Read the model definition and answer for the solid it produces. Units are mm, in the model's axes. A direction names the side the tool comes from. Coordinates: 2 decimals unless noted, no trailing zeros. Loops run counter-clockwise (first coordinate to the right, second up) from the corner with the lowest first, then second, coordinate; pieces in that order, holes last.
from build123d import *

# Parameters (mm, degrees)
ESBO_O1_W                = 400
ESBO_O1_H                = 150
RESSALTO_EXTRUS_O1_DEPTH = 9
ESBO_O2_W                = 10
ESBO_O2_H                = 150
RESSALTO_EXTRUS_O2_DEPTH = 450
ESBO_O5_R                = 35
CORTE_EXTRUS_O1_DEPTH    = 300
ESBO_O6_W                = 400
ESBO_O6_H                = 10
RESSALTO_EXTRUS_O4_DEPTH = 230
ESBO_O8_W                = 100
ESBO_O8_H                = 50
RESSALTO_EXTRUS_O5_DEPTH = 25
ESBO_O9_R                = 5
CORTE_EXTRUS_O3_DEPTH    = 50
ESBO_O7_R                = 5
CORTE_EXTRUS_O2_DEPTH    = 150
ESBO_O11_W               = 100
ESBO_O11_H               = 50
RESSALTO_EXTRUS_O6_DEPTH = 50
ESBO_O12_R               = 5
CORTE_EXTRUS_O4_DEPTH    = 30
ESBO_O13_W               = 44
ESBO_O13_H               = 45
ESBO_O13_H_2             = 44
CORTE_EXTRUS_O5_DEPTH    = 100
ESBO_O14_R               = 5
CORTE_EXTRUS_O6_DEPTH    = 10


with BuildPart() as part:
    # Esboço1 → Ressalto-extrusão1 (new body)
    with BuildSketch(Plane(origin=(0, 0, 0), x_dir=(1, 0, 0), z_dir=(0, 1, 0))):
        Rectangle(ESBO_O1_W, ESBO_O1_H)
    extrude(amount=RESSALTO_EXTRUS_O1_DEPTH)

    # Esboço2 → Ressalto-extrusão2 (add)
    with BuildSketch(Plane(origin=(0, 9, 0), x_dir=(1, 0, 0), z_dir=(0, 1, 0))):
        with Locations((-126, 0)):
            Rectangle(ESBO_O2_W, ESBO_O2_H)
        with Locations((126, 0)):
            Rectangle(ESBO_O2_W, ESBO_O2_H)
    extrude(amount=RESSALTO_EXTRUS_O2_DEPTH)

    # Esboço5 → Corte-extrusão1 (cut)
    with BuildSketch(Plane.ZY.offset(131)):
        with Locations((0, 359)):
            Circle(ESBO_O5_R)
    extrude(amount=-CORTE_EXTRUS_O1_DEPTH, mode=Mode.SUBTRACT)

    # Esboço6 → Ressalto-extrusão4 (add)
    with BuildSketch(Plane.XZ):
        with Locations((0, 80)):
            Rectangle(ESBO_O6_W, ESBO_O6_H)
    extrude(amount=-RESSALTO_EXTRUS_O4_DEPTH)

    # Esboço8 → Ressalto-extrusão5 (add, symmetric)
    with BuildSketch(Plane.ZY):
        with Locations((135, 204)):
            Rectangle(ESBO_O8_W, ESBO_O8_H)
    extrude(amount=RESSALTO_EXTRUS_O5_DEPTH, both=True)

    # Esboço9 → Corte-extrusão3 (cut)
    with BuildSketch(Plane(origin=(0, 230, 0), x_dir=(-1, 0, 0), z_dir=(0, 1, 0))):
        with Locations(Location((0, 155, 0), (0, 0, 90))):
            Circle(ESBO_O9_R)
    extrude(amount=-CORTE_EXTRUS_O3_DEPTH, mode=Mode.SUBTRACT)

    # Esboço7 → Corte-extrusão2 (cut)
    with BuildSketch(Plane(origin=(0, 0, 75), x_dir=(-1, 0, 0), z_dir=(0, 0, -1))):
        with Locations((0, 115)):
            Circle(ESBO_O7_R)
    extrude(amount=-CORTE_EXTRUS_O2_DEPTH, mode=Mode.SUBTRACT)

    # Esboço11 → Ressalto-extrusão6 (add)
    with BuildSketch(Plane.ZY.offset(-75)):
        with Locations((135, 26)):
            Rectangle(ESBO_O11_W, ESBO_O11_H)
    extrude(amount=RESSALTO_EXTRUS_O6_DEPTH)

    # Esboço12 → Corte-extrusão4 (cut)
    with BuildSketch(Plane.ZY.offset(-25)):
        with Locations((139.811131484, 26)):
            Circle(ESBO_O12_R)
    extrude(amount=-CORTE_EXTRUS_O4_DEPTH, mode=Mode.SUBTRACT)

    # Esboço13 → Corte-extrusão5 (cut)
    with BuildSketch(Plane.XY.offset(185)):
        with Locations((50, 25.5)):
            Rectangle(ESBO_O13_W, ESBO_O13_H)
        with Locations((0, 204)):
            Rectangle(ESBO_O13_W, ESBO_O13_H_2)
    extrude(amount=-CORTE_EXTRUS_O5_DEPTH, mode=Mode.SUBTRACT)

    # Esboço14 → Corte-extrusão6 (cut)
    with BuildSketch(Plane.XY.offset(85)):
        with Locations((0, 204)):
            Circle(ESBO_O14_R)
        with Locations((50, 25.5)):
            Circle(ESBO_O14_R)
    extrude(amount=-CORTE_EXTRUS_O6_DEPTH, mode=Mode.SUBTRACT)


solid = part.part
Item 1: A cutting plane is placed at A-A on y = 387. Determine the outline of the cut face in (x, z), then the cut area to 3 significant figures.
Numbers:
outline: (-131, -75) - (-121, -75) - (-121, -21) - (-131, -21) - close; (-131, 21) - (-121, 21) - (-121, 75) - (-131, 75) - close; (121, -75) - (131, -75) - (131, -21) - (121, -21) - close; (121, 21) - (131, 21) - (131, 75) - (121, 75) - close
area: 2,160 mm2
Item 2: Which of the six approach directions +Z, -Z, +X, -X, +Y, -Y give full straight-line access (tool end or side, diameter ignored) to faces 4 (the face through (-25, 204, 134)), 5 (the face through (0, 182, 136)), 6 (the face through (-2, 93, 75))?
Numbers:
face 4: +Z, -X, +Y, -Y
face 5: +Z
face 6: -Z, +Y
Item 3: A cutting plane is placed at B-B on z = 0. Determine the outline of the cut face in (x, y).
Numbers:
outline: (-200, 0) - (200, 0) - (200, 9) - (131, 9) - (131, 324) - (121, 324) - (121, 9) - (-121, 9) - (-121, 324) - (-131, 324) - (-131, 9) - (-200, 9) - close; (-131, 394) - (-121, 394) - (-121, 459) - (-131, 459) - close; (121, 394) - (131, 394) - (131, 459) - (121, 459) - close
Item 4: A cutting plane is placed at C-C on x = 37. Determine the outline of the cut face in (y, z).
Numbers:
outline: (0, -75) - (9, -75) - (9, 75) - (230, 75) - (230, 85) - (51, 85) - (51, 185) - (48, 185) - (48, 85) - (3, 85) - (3, 185) - (1, 185) - (1, 85) - (0, 85) - close
Item 5: A cutting plane is placed at D-D on y = 37. Determine the outline of the cut face in (x, z).
Numbers:
outline: (-200, 75) - (-131, 75) - (-131, -75) - (-121, -75) - (-121, 75) - (121, 75) - (121, -75) - (131, -75) - (131, 75) - (200, 75) - (200, 85) - (75, 85) - (75, 185) - (72, 185) - (72, 85) - (28, 85) - (28, 185) - (25, 185) - (25, 85) - (-200, 85) - close
Item 6: Given pin 1 (12 mm diameter, centred on x = 143, z = 33.5, fed in from +Y); pin 2 (25 mm diameter, centred on x = -9.5, z = 157.5, fed in from +Y); pin 3 (12 mm diameter, centred on x = -49, y = 186.5, fed in from -Z); pin 4 (12 mm diameter, centred on x = -22.5, z = 52, fed in from -Y), each flat-ended and moving along its own axis, determine where each tip first touches the part or whether it passes through.
Numbers:
pin 1: stops at y = 9
pin 2: stops at y = 229
pin 3: stops at z = 75
pin 4: stops at y = 0
Item 7: Find the intervals of material crossed by line 1 along Y through (x, z) = (0, 81); line 2 along X through (y, z) = (119, -4); line 3 along X through (y, z) = (210, 124.5), in increasing order.
Numbers:
line 1: y = 0 to 110, 120 to 199, 209 to 230
line 2: x = -131 to -121, 121 to 131
line 3: x = -25 to -22, 22 to 25
Item 8: Determine the mould class of faces 1 (the face through (-3, 230, 80)), 2 (the face through (-126, 343, 75)), 3 (the face through (50, 3, 136)) for opening direction Y: released by +Y, released by -Y, zero draft, split by the parting line, or undercut.
Numbers:
face 1: released by +Y
face 2: zero draft
face 3: undercut
